Could you check a few things on this model? Use its own coordinates, in mm. A direction names the side the tool comes from. Coordinates: 2 decimals unless noted, no trailing zeros. Loops run counter-clockwise (first coordinate to the right, second up) from the corner with the lowest first, then second, coordinate; pieces in that order, holes last. Notation, with made-up numbers: (-27.75, -2.75) - (17.25, -2.75) arc R14 ccw to (17.25, 5.25) - close; hole circle Ø7 at (1.5, 22.25). An arc over 180 degrees is marked (long way). Use CSV: the item, a comma, the result in double quotes.
from build123d import *

# Parameters (mm, degrees)
F0_R     = 10
F1_DEPTH = 30
F2_R     = 8
F3_DEPTH = 20
F4_R     = 4
F5_DEPTH = 30.001
F7_DEPTH = 5


with BuildPart() as f1:
    # F0 (on Front) → F1 (new body)
    with BuildSketch(Plane.XZ):
        Circle(F0_R)
    extrude(amount=F1_DEPTH)

    # F2 (on face) → F3 (cut)
    with BuildSketch(Plane.XZ.offset(30)):
        Circle(F2_R)
    extrude(amount=-F3_DEPTH, mode=Mode.SUBTRACT)

    # F4 (on face) → F5 (cut, through all)
    with BuildSketch(Plane(origin=(0, 0, 0), x_dir=(-1, 0, 0), z_dir=(0, 1, 0))):
        Circle(F4_R)
    extrude(amount=-F5_DEPTH, mode=Mode.SUBTRACT)

    # F6 (on face) → F7 (cut)
    with BuildSketch(Plane(origin=(0, 0, 0), x_dir=(-1, 0, 0), z_dir=(0, 1, 0))):
        Polygon((4.846734, 4.950674), (-1.864042, 6.672732), (-6.710776, 1.722058), (-4.846734, -4.950674), (1.864042, -6.672732), (6.710776, -1.722058), align=None)
    extrude(amount=-F7_DEPTH, mode=Mode.SUBTRACT)


solid = f1.part
(1) Will these pins go through, and if not, where does the flat tip stop? pin 1 (9.5 mm diameter, centred on x = 0, z = 0, fed in from -Y); pin 2 (4 mm diameter, centred on x = 7.5, y = -27, fed in from -Z); pin 3 (5 mm diameter, centred on x = 3, y = -12.5, fed in from +Z).
Computed:
pin 1,"stops at y = -10"
pin 2,"stops at z = -8.35"
pin 3,"stops at z = 9.99"
(2) Suppose I cut it at C-C (z = 0). Write out the boundary of the cut face in (x, y), plus the area to 3 significant figures.
Computed:
outline,"(-10, -30) - (-8, -30) - (-8, -10) - (-4, -10) - (-4, -5) - (-6.23, -5) - (-6.23, 0) - (-10, 0) - close; (4, -10) - (8, -10) - (8, -30) - (10, -30) - (10, 0) - (6.23, 0) - (6.23, -5) - (4, -5) - close"
area,"178 mm²"
(3) Suppose I cut it at A-A (x = 3.25). Write out the boundary of the cut face in (y, z), plus the area to 3 significant figures.
Computed:
outline,"(-30, -9.46) - (0, -9.46) - (0, -5.36) - (-5, -5.36) - (-5, -2.33) - (-10, -2.33) - (-10, -7.31) - (-30, -7.31) - close; (-30, 7.31) - (-10, 7.31) - (-10, 2.33) - (-5, 2.33) - (-5, 5.26) - (0, 5.26) - (0, 9.46) - (-30, 9.46) - close"
area,"199 mm²"
(4) Suppose I cut it at D-D (z = 6). Write out the boundary of the cut face in (x, y).
Computed:
outline,"(-8, -30) - (-5.29, -30) - (-5.29, -10) - (5.29, -10) - (5.29, -30) - (8, -30) - (8, 0) - (2.52, 0) - (2.52, -5) - (-0.76, -5) - (-0.76, 0) - (-8, 0) - close"
(5) Thinking about a two-plate mould opening in X: for faces 4 (the face through (-2.17, -14.79, -9.76)), 5 (the face through (1.54, -2.46, -5.8)), 6 (the face through (0, -30, 8.2)), which applies, +X half, -X half, draft (parallel to the pull), parting line (faces both ways), or undercut?
Computed:
face 4,"parting line"
face 5,"undercut"
face 6,"draft"
(6) Please list where these lines run through material, in increasing order: line 1 (Z direction, x = 0, y = -7.75); line 2 (Z direction, x = 0, y = -18.5); line 3 (X direction, y = -27, z = 3).
Computed:
line 1,"z = -10 to -4, 4 to 10"
line 2,"z = -10 to -8, 8 to 10"
line 3,"x = -9.54 to -7.42, 7.42 to 9.54"
(7) Which directions (+Z, -Z, +X, -X, +Y, -Y) give clear straight access to the entire face, cutting with the end or side of a thin tool? Please do faces 1 (the face through (-3, -5, -3)), 2 (the face through (0.867, -7.465, -3.905)), 3 (the face through (-1.73, -20.14, -7.81)).
Computed:
face 1,"+Y"
face 2,"+Y, -Y"
face 3,"-Y"
(8) Suppose I cut it at B-B (y = -3). Write out the boundary of the cut face in (x, z), plus the area to 3 significant figures.
Computed:
outline,"circle Ø20 at (0, 0); hole (-6.71, -1.72) - (-1.86, -6.67) - (4.85, -4.95) - (6.71, 1.72) - (1.86, 6.67) - (-4.85, 4.95) - close"
area,"189 mm²"
